Can you work these out from the drawing? Everything is in mm from the part's minimum corner. A direction names the side the tool comes from. Round coordinates to 2 decimals unless told otherwise and drop trailing zeros. Write each loop counter-clockwise with the first axis right and the second up, starting at its lowest first coordinate (ties: lowest second). Pieces come first, ordered by that corner, then holes. Notation, with made-up numbers: (14, 54) - (36, 54) arc R26 cw to (36, 73) - close; hole circle Ø9 at (19.25, 25.25). An arc over 180 degrees is marked (long way). One line per item, written item: value. Start each with the question number.
(1) If I drill on L1, parallel to Y at x = 20, z = 10.25; L2, parallel to Z at x = 20, y = 7.25; L3, parallel to Y at x = 18, z = 12.5, over which ranges is the centre line in solid material (lowest first)? Write a range as from..to.
(2) I want a section at B-B on y = 5.75. List the corners of the cut face in (x, z) for me, plus the area to 3 significant figures.
(3) I'm going to push a flat-ended pin straight in: pin 1 Ø4.5 at (x, y) = (13, 7) entering from +Z. Where does the tip first touch, or does it pass through?
(4) I want a section at A-A on x = 5.1. List the corners of the cut face in (y, z) for me, plus the area to 3 significant figures.
(5) I want a section at D-D on x = 21. List the corners of the cut face in (y, z) for me.
(6) I want a section at C-C on z = 4. List the corners of the cut face in (x, y) for me.
(7) Thinking about a two-plate mould opening in Y: for the marked faces 1, 2 and 3, which applies, +Y half, -Y half, draft (parallel to the pull), parting line (faces both ways), or undercut?
(8) On a 3-axis mill with a long thin cutter (end or side, diameter ignored), from which of +Z, -Z, +X, -X, +Y, -Y can I reach the whole of each face in a straight line? I mean the marked faces 4, 5 and 6. Say none if no direction works.
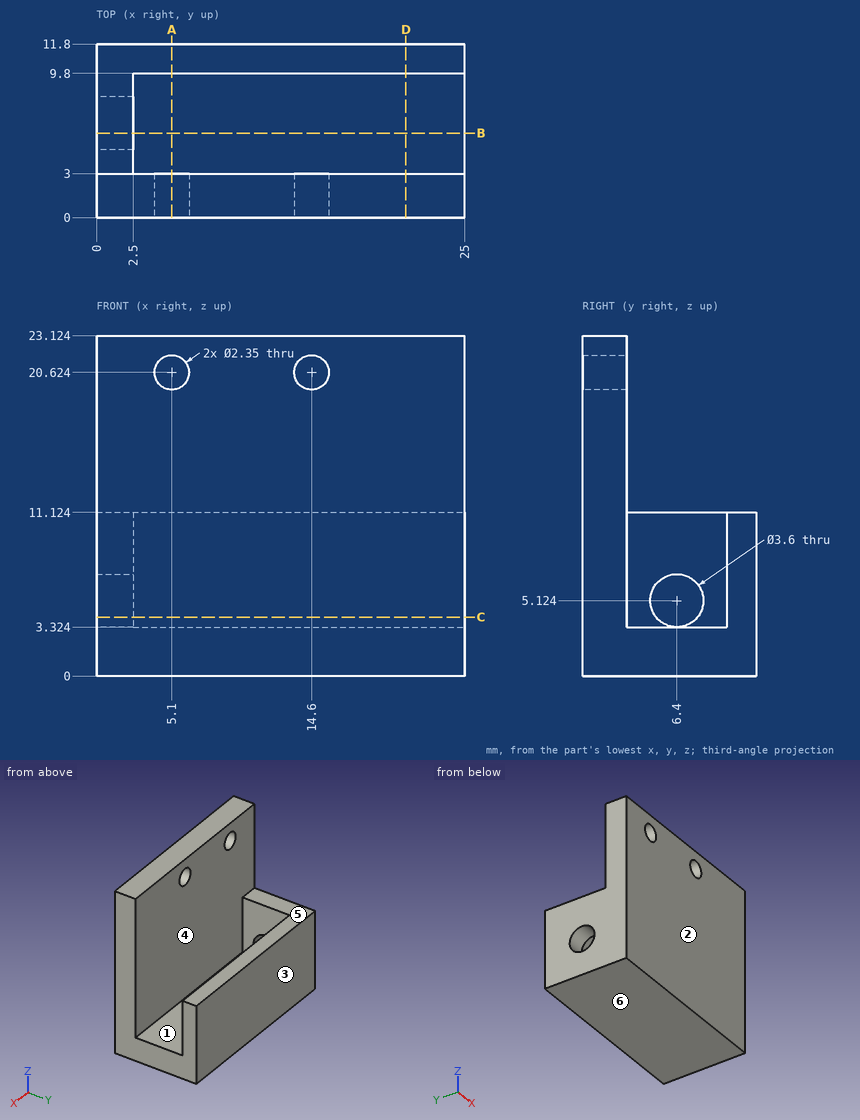
Established:
1. L1: 0..3, 9.8..11.8
1. L2: 0..3.32
1. L3: 0..3
2. outline: (0, 0) - (25, 0) - (25, 3.32) - (2.5, 3.32) - (2.5, 3.45) - (0, 3.45) - close; (0, 6.8) - (2.5, 6.8) - (2.5, 11.12) - (0, 11.12) - close
2. area: 94.2 mm2
3. pin 1: z = 3.32
4. outline: (0, 0) - (11.8, 0) - (11.8, 11.12) - (9.8, 11.12) - (9.8, 3.32) - (3, 3.32) - (3, 19.45) - (0, 19.45) - close; (0, 21.8) - (3, 21.8) - (3, 23.12) - (0, 23.12) - close
4. area: 107 mm2
5. outline: (0, 0) - (11.8, 0) - (11.8, 11.12) - (9.8, 11.12) - (9.8, 3.32) - (3, 3.32) - (3, 23.12) - (0, 23.12) - close
6. outline: (0, 0) - (25, 0) - (25, 3) - (2.5, 3) - (2.5, 4.99) - (0, 4.99) - close; (0, 7.81) - (2.5, 7.81) - (2.5, 9.8) - (25, 9.8) - (25, 11.8) - (0, 11.8) - close
7. face 1: undercut
7. face 2: -Y half
7. face 3: +Y half
8. face 4: +Z, +X
8. face 5: +Z, +X, -X, +Y
8. face 6: -Z, +X, -X, +Y, -Y
